from build123d import *

# Parameters (mm, degrees)
BOSS_EXTRUDE1_DEPTH = 15


with BuildPart() as part:
    # Sketch1 → Boss-Extrude1 (new body)
    with BuildSketch(Plane(origin=(0, 0, 0), x_dir=(1, 0, 0), z_dir=(0, 1, 0))):
        with BuildLine():
            Line((0, 75), (0, 60))
            ThreePointArc((0, 60), (20.5212086, 56.381557247), (38.567256581, 45.962666587))
            Line((38.567256581, 45.962666587), (48.209070726, 57.453333234))
            ThreePointArc((48.209070726, 57.453333234), (25.651510749, 70.476946559), (0, 75))
        make_face()
        with BuildLine():
            Line((48.209070726, 57.453333234), (38.567256581, 45.962666587))
            Line((38.567256581, 45.962666587), (48.066207676, 37.992100227))
            Line((48.066207676, 37.992100227), (57.044556278, 48.692079429))
            ThreePointArc((57.044556278, 48.692079429), (52.808819258, 53.256254173), (48.209070726, 57.453333234))
        make_face()
        with BuildLine():
            Line((57.708021821, 49.482766874), (48.209070726, 57.453333234))
            ThreePointArc((48.209070726, 57.453333234), (52.808819258, 53.256254173), (57.044556278, 48.692079429))
            Line((57.044556278, 48.692079429), (57.708021821, 49.482766874))
        make_face()
        with BuildLine():
            ThreePointArc((-12.4, 73.967830846), (-6.22144222, 74.741512272), (0, 75))
            Line((0, 75), (-12.4, 75))
            Line((-12.4, 75), (-12.4, 73.967830846))
        make_face()
        with BuildLine():
            Line((-12.4, 60), (0, 60))
            Line((0, 60), (0, 75))
            ThreePointArc((0, 75), (-6.22144222, 74.741512272), (-12.4, 73.967830846))
            Line((-12.4, 73.967830846), (-12.4, 60))
        make_face()
    extrude(amount=BOSS_EXTRUDE1_DEPTH)


solid = part.part
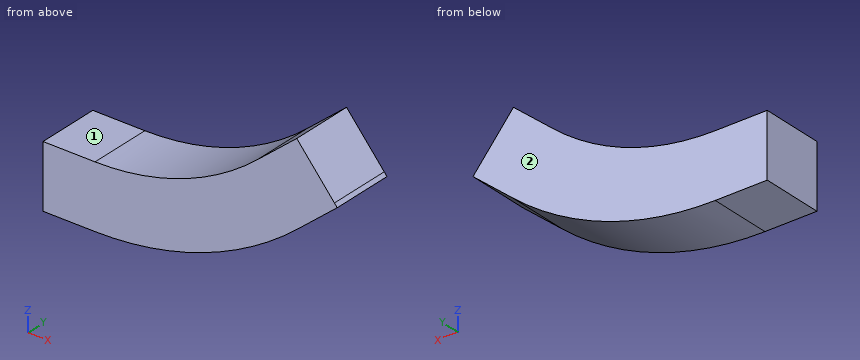
Input: part model. Units: mm. Frame: model coordinates. Face numbers are marked on the shaded views. A direction names the side the tool comes from. Coordinates: 2 decimals unless noted, no trailing zeros. Order: outer loops, then holes, each group sorted by start corner. A loop starts at its lowest first (then second) coordinate and runs counter-clockwise, first axis right, second up. Notation, with made-up numbers: M 44,85 L 87,85 A26 ccw 87,109 Z; hole C 80.5,7 d10. An arc over 180 degrees is marked long. Answer as CSV lines item,"result".
1. Section B-B (x = -4). Return the cut outline in (y, z), then the cut area to 3 significant figures.
Reported:
outline,"M 0,-75 L 15,-75 L 15,-60 L 0,-60 Z"
area,"225 mm2"
2. Section C-C (z = -48). Return the cut outline in (x, y), then the cut area to 3 significant figures.
Reported:
outline,"M 36,0 L 56.46,0 L 56.46,15 L 36,15 Z"
area,"307 mm2"
3. First-contact query: P1, Ø2, axis at x = 30, y = 7.5, coming from the -Z side; P2, Ø6, axis at x = 31, y = 8, coming from the +Z side; P3, Ø8, axis at x = -1, y = 3, coming from the +Z side; P4, Ø10, axis at x = 10, z = -68, coming from the -Y side. Flat tips, straight axial feed; report the tip coordinate or a pass-through.
Reported:
P1,"z = -69.17"
P2,"z = -49.44"
P3,"z = -59.92"
P4,"y = 0"
4. Section A-A (y = 7). Return the cut outline in (x, z), then the cut area to 3 significant figures.
Reported:
outline,"M -12.4,-75 L 0,-75 A75 ccw 48.21,-57.45 L 57.71,-49.48 L 48.07,-37.99 L 38.57,-45.96 A60 cw 0,-60 L -12.4,-60 Z"
area,"1,080 mm2"
5. Access query for the marked faces 1 and 2. Directions: +Z, -Z, +X, -X, +Y, -Y. A direction counts if a zero-diameter tool reaches every point of the face in a straight line with its end or side. Return the directions, or none.
Reported:
face 1,"+Z, -X, +Y, -Y"
face 2,"+Z, -Z, +X, -X, +Y"
6. Material intervals for line 1 (Z direction, x = -6, y = 13.75); line 2 (X direction, y = 2, z = -54); line 3 (Z direction, x = 53.5, y = 10.75), sorted ascending. Write a range as from..to.
Reported:
line 1,"-75..-60"
line 2,"26.15..52.32"
line 3,"-53.01..-44.47"
